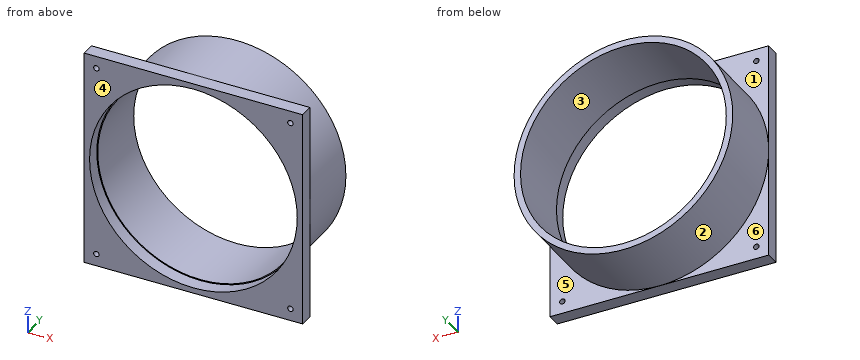
```python
from build123d import *

# Parameters (mm, degrees)
F0_W     = 80
F0_H     = 80
F0_R     = 1
F0_R_2   = 38
F1_DEPTH = 2.5
F3_R     = 40
F3_R_2   = 37.6432669416
F4_DEPTH = 24.8567536473


with BuildPart() as f1:
    # F0 (on Front) → F1 (new body, symmetric)
    with BuildSketch(Plane.XZ):
        Rectangle(F0_W, F0_H)
        with Locations((-35.5, -35.5)):
            Circle(F0_R, mode=Mode.SUBTRACT)
        with Locations((35.5, -35.5)):
            Circle(F0_R, mode=Mode.SUBTRACT)
        with Locations((-35.5, 35.5)):
            Circle(F0_R, mode=Mode.SUBTRACT)
        Circle(F0_R_2, mode=Mode.SUBTRACT)
        with Locations((35.5, 35.5)):
            Circle(F0_R, mode=Mode.SUBTRACT)
    extrude(amount=F1_DEPTH, both=True)

    # F3 (on face) → F4 (join)
    with BuildSketch(Plane(origin=(0, 2.5, 0), x_dir=(-1, 0, 0), z_dir=(0, 1, 0))):
        Circle(F3_R)
        Circle(F3_R_2, mode=Mode.SUBTRACT)
    extrude(amount=F4_DEPTH)


solid = f1.part
```
Read the model definition and answer for the solid it produces. Units are mm, in the model's axes. Face numbers are marked on the shaded views. A direction names the side the tool comes from. Round coordinates to 2 decimals unless told otherwise and drop trailing zeros. Write each loop counter-clockwise with the first axis right and the second up, starting at its lowest first coordinate (ties: lowest second). Pieces come first, ordered by that corner, then holes. Notation, with made-up numbers: (-29.75, 84) - (21.25, 84) arc R9 ccw to (21.25, 91) - close; hole circle Ø1 at (83, 52). An arc over 180 degrees is marked (long way). One line per item, written item: value.
Q1. Each of these flat-tipped pins is pushed along its axis until it touches: P1, Ø2, axis at x = 16.5, y = 5.5, coming from the -Z side; P2, Ø2.5, axis at x = 35.5, z = 35.5, coming from the +Y side; P3, Ø1.5, axis at x = 8, y = 7, coming from the -Z side. Where does it stop, or does it pass through?
The answers:
P1: stops at z = -36.87
P2: stops at y = 2.5
P3: stops at z = -39.34
Q2. Find section B-B (z = -29). Determine the outline of the cut face in (x, y).
The answers:
outline: (-40, -2.5) - (-24.56, -2.5) - (-24.56, 2.5) - (-24, 2.5) - (-24, 27.36) - (-27.55, 27.36) - (-27.55, 2.5) - (-40, 2.5) - close; (24, 2.5) - (24.56, 2.5) - (24.56, -2.5) - (40, -2.5) - (40, 2.5) - (27.55, 2.5) - (27.55, 27.36) - (24, 27.36) - close
Q3. Find section A-A (x = 2). Determine the outline of the cut face in (y, z), and give its area (3 significant figures).
The answers:
outline: (-2.5, -40) - (2.5, -40) - (2.5, -39.95) - (27.36, -39.95) - (27.36, -37.59) - (2.5, -37.59) - (2.5, -37.95) - (-2.5, -37.95) - close; (-2.5, 37.95) - (2.5, 37.95) - (2.5, 37.59) - (27.36, 37.59) - (27.36, 39.95) - (2.5, 39.95) - (2.5, 40) - (-2.5, 40) - close
area: 138 mm2
Q4. Find section C-C (x = 35.5). Determine the outline of the cut face in (y, z).
The answers:
outline: (-2.5, -40) - (2.5, -40) - (2.5, -36.5) - (-2.5, -36.5) - close; (-2.5, -34.5) - (2.5, -34.5) - (2.5, -18.43) - (27.36, -18.43) - (27.36, -12.52) - (2.5, -12.52) - (2.5, -13.56) - (-2.5, -13.56) - close; (-2.5, 13.56) - (2.5, 13.56) - (2.5, 12.52) - (27.36, 12.52) - (27.36, 18.43) - (2.5, 18.43) - (2.5, 34.5) - (-2.5, 34.5) - close; (-2.5, 36.5) - (2.5, 36.5) - (2.5, 40) - (-2.5, 40) - close
Q5. Which of the six approach directions +Z, -Z, +X, -X, +Y, -Y give full straight-line access (tool end or side, diameter ignored) to the marked faces 4, 5 and 6?
The answers:
face 4: +Z, -Z, +X, -X, -Y
face 5: -Z, +X, +Y
face 6: -Z, -X, +Y
Q6. Straight lines are drawn through the part: line 1 (X direction, y = 1, z = 5); line 2 (X direction, y = 18, z = -30.5); line 3 (Z direction, x = -18, y = 8.5). For each, find the intervals that lie inside material, in ascending order. Write a range as from..to.
The answers:
line 1: x = -40..-37.67, 37.67..40
line 2: x = -25.88..-22.06, 22.06..25.88
line 3: z = -35.72..-33.06, 33.06..35.72
Q7. Find section D-D (y = 25). Determine the outline of the cut face in (x, z).
The answers:
outline: circle Ø80 at (0, 0); hole circle Ø75.29 at (0, 0)
Q8. For a pull along X with two mould halves and no side action, classify the marked faces 1, 2 and 3 as pulls with the +X half, pulls with the -X half, needs draft (parallel to the pull), parting line crosses it, or undercut.
The answers:
face 1: needs draft
face 2: parting line crosses it
face 3: undercut
